Work out the finished part from the listing and answer in its coordinate system (mm). A direction names the side the tool comes from. Coordinates: 2 decimals unless noted, no trailing zeros. Write each loop counter-clockwise with the first axis right and the second up, starting at its lowest first coordinate (ties: lowest second). Pieces come first, ordered by that corner, then holes. Notation, with made-up numbers: M 53.5,-11.75 L 74.5,-11.75 A19 ccw 74.5,20.25 Z; hole C 47,82.25 d1. An arc over 180 degrees is marked long. Answer as CSV lines item,"result". Start each with the question number.
(1) A cutting plane is placed at B-B on x = 12. Give the vertices of the cut face in (y, z).
(2) Find the intervals of material crossed by L1, parallel to Y at x = 160.5, z = 6.5; L2, parallel to X at y = 14.5, z = 7.25; L3, parallel to Y at x = 116.5, z = 11.25, in increasing order. Write a range as [from, to].
(3) The mould has two halves that part along X. Classify faces 1 (the flat face through (113.877, 8, 8)), 2 (the flat face through (164, 50.8, 8)), 3 (the flat face through (15.24, 89, 8)): released by +X, released by -X, zero draft, split by the parting line, or undercut.
(4) A cutting plane is placed at C-C on z = 3. Give the vertices of the cut face in (x, y).
(5) A cutting plane is placed at D-D on y = 12. Give the vertices of the cut face in (x, z), then the cut area to 3 significant figures.
(6) For faces 4 (the flat face through (15.24, 38, 8)), 5 (the flat face through (164, 76.2, 8)), 6 (the flat face through (171.45, 63, 8)), determine the directions among +Z, -Z, +X, -X, +Y, -Y from which every point of the face is accessible in a straight line to the end or side of a thin tool.
(7) A cutting plane is placed at A-A on y = 63.5. Give the vertices of the cut face in (x, z).
(8) Flat-ended cylindrical pins translate along their axes: P1, Ø1, axis at y = 114, z = 4.5, coming from the -X side; P2, Ø13.5, axis at x = 61.976, y = 63.5, coming from the +Z side; P3, Ø4.5, axis at y = 39, z = 8, coming from the +X side; P4, Ø2, axis at y = 47.5, z = 3.5, coming from the -X side. Find the tip coordinate at first contact, or state that the pin passes through.
from build123d import *

# Parameters (mm, degrees)
SKETCH1_W           = 171.45
SKETCH1_H           = 127
BOSS_EXTRUDE1_DEPTH = 15.24
SKETCH5_W           = 15.24
SKETCH5_H           = 25.4
CUT_EXTRUDE1_DEPTH  = 15.24
SKETCH11_R          = 11.43
CUT_EXTRUDE3_DEPTH  = 15.24
SKETCH7_W           = 21.166666666
SKETCH7_H           = 15.24
CUT_EXTRUDE4_DEPTH  = 15.24


with BuildPart() as part:
    # Sketch1 → Boss-Extrude1 (new body)
    with BuildSketch(Plane.XY):
        with Locations((85.725, 63.5)):
            Rectangle(SKETCH1_W, SKETCH1_H)
    extrude(amount=BOSS_EXTRUDE1_DEPTH)

    # Sketch5 → Cut-Extrude1 (cut)
    with BuildSketch(Plane.XY.offset(15.24)):
        with Locations((7.62, 88.9)):
            Rectangle(SKETCH5_W, SKETCH5_H)
        with Locations((7.62, 38.1)):
            Rectangle(SKETCH5_W, SKETCH5_H)
        with Locations((163.83, 88.9)):
            Rectangle(SKETCH5_W, SKETCH5_H)
        with Locations((163.83, 38.1)):
            Rectangle(SKETCH5_W, SKETCH5_H)
    extrude(amount=-CUT_EXTRUDE1_DEPTH, mode=Mode.SUBTRACT)

    # Sketch11 → Cut-Extrude3 (cut)
    with BuildSketch(Plane.XY.offset(15.24)):
        with Locations((61.976, 63.5)):
            Circle(SKETCH11_R)
    extrude(amount=-CUT_EXTRUDE3_DEPTH, mode=Mode.SUBTRACT)

    # Sketch7 → Cut-Extrude4 (cut)
    with BuildSketch(Plane.XY.offset(15.24)):
        with Locations((124.46, 7.62)):
            Rectangle(SKETCH7_W, SKETCH7_H)
    extrude(amount=-CUT_EXTRUDE4_DEPTH, mode=Mode.SUBTRACT)


solid = part.part
Here are the results:
1,outline,"M 0,0 L 25.4,0 L 25.4,15.24 L 0,15.24 Z; M 50.8,0 L 76.2,0 L 76.2,15.24 L 50.8,15.24 Z; M 101.6,0 L 127,0 L 127,15.24 L 101.6,15.24 Z"
2,L1,"y = [0, 25.4], [50.8, 76.2], [101.6, 127]"
2,L2,"x = [0, 113.88], [135.04, 171.45]"
2,L3,"y = [15.24, 127]"
3,face 1,"undercut"
3,face 2,"zero draft"
3,face 3,"released by -X"
4,outline,"M 0,0 L 113.88,0 L 113.88,15.24 L 135.04,15.24 L 135.04,0 L 171.45,0 L 171.45,25.4 L 156.21,25.4 L 156.21,50.8 L 171.45,50.8 L 171.45,76.2 L 156.21,76.2 L 156.21,101.6 L 171.45,101.6 L 171.45,127 L 0,127 L 0,101.6 L 15.24,101.6 L 15.24,76.2 L 0,76.2 L 0,50.8 L 15.24,50.8 L 15.24,25.4 L 0,25.4 Z; hole C 61.98,63.5 d22.86"
5,outline,"M 0,0 L 113.88,0 L 113.88,15.24 L 0,15.24 Z; M 135.04,0 L 171.45,0 L 171.45,15.24 L 135.04,15.24 Z"
5,area,"2,290 mm^2"
6,face 4,"+Z, -Z, -X"
6,face 5,"+Z, -Z, +X"
6,face 6,"+Z, -Z, +X, +Y, -Y"
7,outline,"M 0,0 L 50.55,0 L 50.55,15.24 L 0,15.24 Z; M 73.41,0 L 171.45,0 L 171.45,15.24 L 73.41,15.24 Z"
8,P1,"stops at x = 0"
8,P2,"passes through"
8,P3,"stops at x = 156.21"
8,P4,"stops at x = 15.24"
